Source: three-view drawing plus pictorial views. Frame: mm from the lowest corner of the part. Round coordinates to 2 decimals unless told otherwise and drop trailing zeros. Order: outer loops, then holes, each group sorted by start corner. A loop starts at its lowest first (then second) coordinate and runs counter-clockwise, first axis right, second up. Notation, with made-up numbers: (29, -24.75) - (70, -24.75) arc R24 ccw to (70, -11.75) - close; hole circle Ø5 at (67.5, 23.5). An arc over 180 degrees is marked (long way). Use one line per item in the form item = value. Start each with the question number.
Q1. Cut plane D-D, the plane x = 22. Return the cut outline in (y, z) (1 decimal).
Q2. Cut plane B-B, the plane z = 23.5. Return the cut outline in (x, y).
Q3. Cut plane C-C, the plane y = 1.8. Return the cut outline in (x, z) (1 decimal), and give its area (3 significant figures).
Q4. Ray query, line 1 (Z direction, x = 38.1, y = 0.95) (1 decimal); line 2 (X direction, y = 2.25, z = 31.5) (1 decimal); line 3 (X direction, y = 0.3, z = 16) (1 decimal). Return the intervals inside material, ascending. Write a range as [from, to].
Q5. Cut plane A-A, the plane x = 3.81. Return the cut outline in (y, z) (1 decimal).
Q6. Pin query (flat end, axial travel): pin 1 Ø0.7 at (x, y) = (1, 1.5) entering from -Z. Return the tip coordinate at first contact, or that it passes through.
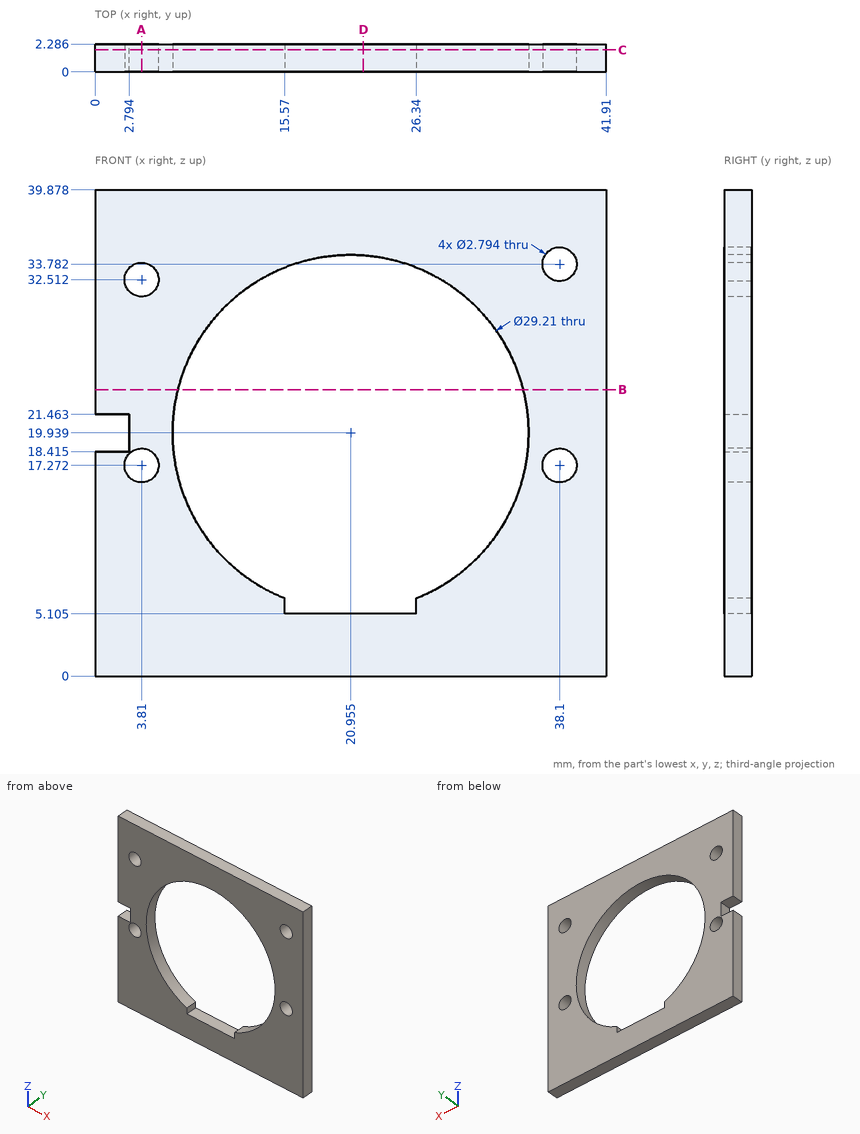
Completed:
q1.outline = (0, 0) - (2.3, 0) - (2.3, 5.1) - (0, 5.1) - close; (0, 34.5) - (2.3, 34.5) - (2.3, 39.9) - (0, 39.9) - close
q2.outline = (0, 0) - (6.79, 0) - (6.79, 2.29) - (0, 2.29) - close; (35.12, 0) - (41.91, 0) - (41.91, 2.29) - (35.12, 2.29) - close
q3.outline = (0, 0) - (41.9, 0) - (41.9, 39.9) - (0, 39.9) - (0, 21.5) - (2.8, 21.5) - (2.8, 18.4) - (0, 18.4) - close; hole circle Ø2.8 at (3.8, 17.3); hole circle Ø2.8 at (3.8, 32.5); hole (15.6, 5.1) - (26.3, 5.1) - (26.3, 6.4) arc R14.6 ccw (long way) to (15.6, 6.4) - close; hole circle Ø2.8 at (38.1, 17.3); hole circle Ø2.8 at (38.1, 33.8)
q3.area = 962 mm2
q4.line_1 = [0, 15.9], [18.7, 32.4], [35.2, 39.9]
q4.line_2 = [0, 2.8], [4.8, 12], [29.9, 41.9]
q4.line_3 = [0, 3.2], [4.4, 6.9], [35, 37.5], [38.7, 41.9]
q5.outline = (0, 0) - (2.3, 0) - (2.3, 15.9) - (0, 15.9) - close; (0, 18.7) - (2.3, 18.7) - (2.3, 31.1) - (0, 31.1) - close; (0, 33.9) - (2.3, 33.9) - (2.3, 39.9) - (0, 39.9) - close
q6.pin_1 = 0
